from build123d import *

# Parameters (mm, degrees)
SKETCH1_W           = 533.4
SKETCH1_H           = 12.7
BOSS_EXTRUDE1_DEPTH = 6.35
SKETCH2_W           = 25.4
SKETCH2_H           = 6.35
CUT_EXTRUDE1_DEPTH  = 7.35
LPATTERN1_COUNT     = 4
LPATTERN1_PITCH     = 133.35


with BuildPart() as part:
    # Sketch1 → Boss-Extrude1 (new body)
    with BuildSketch(Plane(origin=(0, 0, 0), x_dir=(1, 0, 0), z_dir=(0, 1, 0))):
        Rectangle(SKETCH1_W, SKETCH1_H)
    extrude(amount=BOSS_EXTRUDE1_DEPTH)

    # Sketch2 → Cut-Extrude1 (cut, through all)
    with BuildSketch(Plane(origin=(0, 6.35, 0), x_dir=(1, 0, 0), z_dir=(0, 1, 0))):
        with Locations((-200.025, 0)):
            Rectangle(SKETCH2_W, SKETCH2_H)
    cut_extrude1 = extrude(amount=-CUT_EXTRUDE1_DEPTH, mode=Mode.SUBTRACT)

    # LPattern1: Cut-Extrude1 ×4
    with Locations(*[(i * LPATTERN1_PITCH, 0, 0) for i in range(1, LPATTERN1_COUNT)]):
        add(cut_extrude1, mode=Mode.SUBTRACT)


solid = part.part
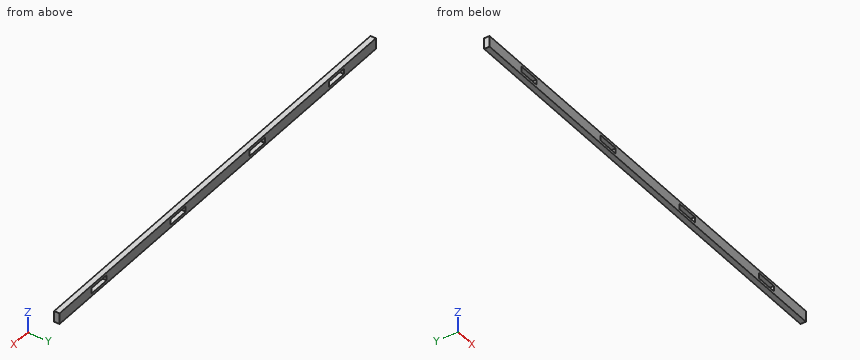
CAD build for the part. Positions are in the model's coordinates, mm. Round coordinates to 2 decimals unless told otherwise and drop trailing zeros. Loops run counter-clockwise (first coordinate to the right, second up) from the corner with the lowest first, then second, coordinate; pieces in that order, holes last. Notation, with made-up numbers: M 18.5,18 L 70.5,18 A6 cw 70.5,26 Z; hole C -4.5,-35.75 d11. An arc over 180 degrees is marked long. One line per question, with ' | ' between items. Start each with the question number.
Item 1: Cut at A-A, the plane x = 58.5. Write the cut outline in (y, z) (3 decimals).
Item 2: Cut at C-C, the plane z = -1.25. Write the cut outline in (x, y) (3 decimals), plus the area to 3 significant figures.
Item 3: Cut at B-B, the plane y = 5. Write the cut outline in (x, z) (3 decimals).
Item 4: Wall check: line 1 (X direction, y = 1, z = 1.5) (3 decimals); line 2 (Z direction, x = -71, y = 2.75) (3 decimals). Give the ranges that are in metal, low to high.
Responses:
1) outline: M 0,-6.35 L 6.35,-6.35 L 6.35,-3.175 L 0,-3.175 Z; M 0,3.175 L 6.35,3.175 L 6.35,6.35 L 0,6.35 Z
2) outline: M -266.7,0 L -212.725,0 L -212.725,6.35 L -266.7,6.35 Z; M -187.325,0 L -79.375,0 L -79.375,6.35 L -187.325,6.35 Z; M -53.975,0 L 53.975,0 L 53.975,6.35 L -53.975,6.35 Z; M 79.375,0 L 187.325,0 L 187.325,6.35 L 79.375,6.35 Z; M 212.725,0 L 266.7,0 L 266.7,6.35 L 212.725,6.35 Z | area: 2,740 mm²
3) outline: M -266.7,-6.35 L 266.7,-6.35 L 266.7,6.35 L -266.7,6.35 Z; hole M -212.725,-3.175 L -187.325,-3.175 L -187.325,3.175 L -212.725,3.175 Z; hole M -79.375,-3.175 L -53.975,-3.175 L -53.975,3.175 L -79.375,3.175 Z; hole M 53.975,-3.175 L 79.375,-3.175 L 79.375,3.175 L 53.975,3.175 Z; hole M 187.325,-3.175 L 212.725,-3.175 L 212.725,3.175 L 187.325,3.175 Z
4) line 1: x = -266.7 to -212.725, -187.325 to -79.375, -53.975 to 53.975, 79.375 to 187.325, 212.725 to 266.7 | line 2: z = -6.35 to -3.175, 3.175 to 6.35
